Design review of the part shown in the three views and the two pictorial views. Dimensions are in mm from the part's minimum x, y and z. A direction names the side the tool comes from. Give positions to 0.01 mm unless a question says otherwise; leave off trailing zeros. Order: outer loops, then holes, each group sorted by start corner. A loop starts at its lowest first (then second) coordinate and runs counter-clockwise, first axis right, second up.
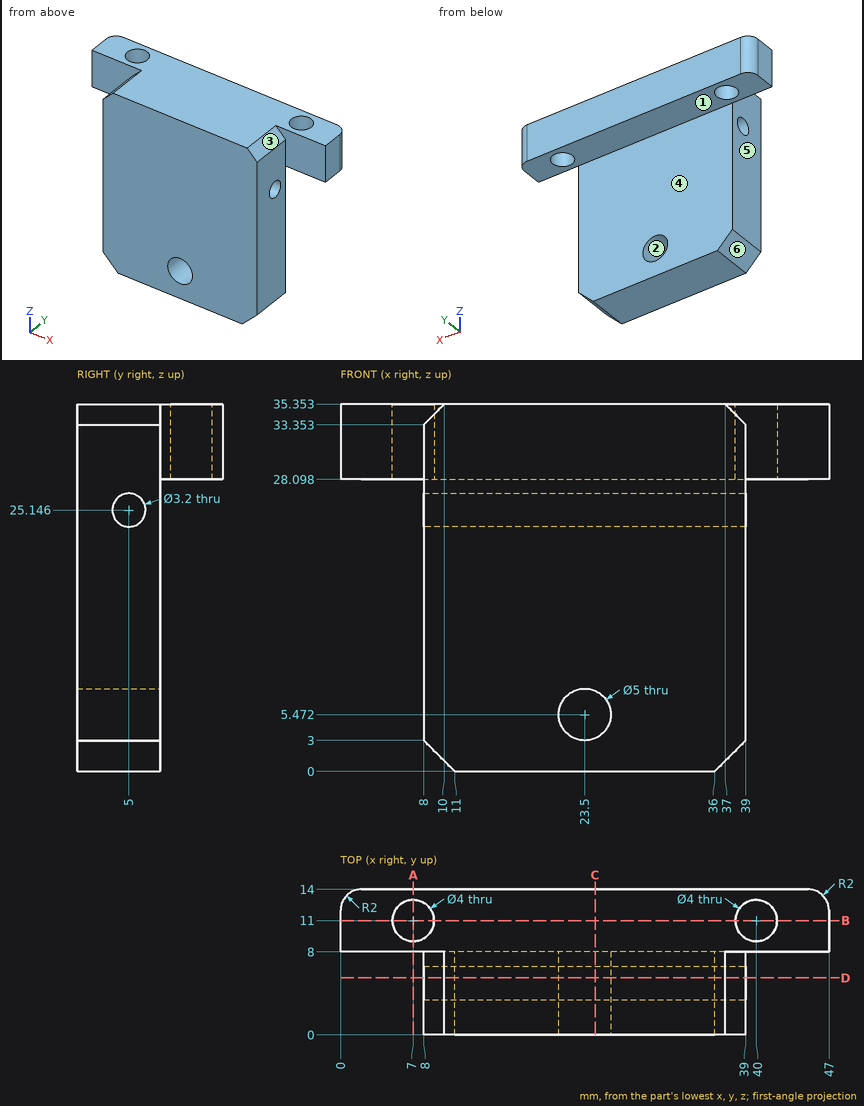
Item 1: Take a section at C-C (x = 24.5). Give the boundary of the cut face in (y, z) (1 decimal).
Values found:
outline: (0, 0) - (8, 0) - (8, 3.2) - (0, 3.2) - close; (0, 7.8) - (8, 7.8) - (8, 28.1) - (14, 28.1) - (14, 35.4) - (0, 35.4) - close; hole circle Ø3.2 at (5, 25.1)
Item 2: Take a section at D-D (y = 5.5). Give the boundary of the cut face in (x, z) (1 decimal).
Values found:
outline: (8, 3) - (11, 0) - (36, 0) - (39, 3) - (39, 23.6) - (8, 23.6) - close; (8, 26.7) - (39, 26.7) - (39, 33.4) - (37, 35.4) - (10, 35.4) - (8, 33.4) - close; hole circle Ø5 at (23.5, 5.5)
Item 3: For the marked faces 4, 5 and 6, list the 3-axis set-ups (+Z, -Z, +X, -X, +Y, -Y) from which the entire face can be reached by the end or side of a thin tool; tool diameter is ignored.
Values found:
face 4: -Z, +X, -X, +Y
face 5: +Z, -Z, -X, -Y
face 6: -Z, -X, +Y, -Y
Item 4: Take a section at A-A (x = 7). Give the boundary of the cut face in (y, z), and give its area (3 significant figures).
Values found:
outline: (8, 28.1) - (9, 28.1) - (9, 35.35) - (8, 35.35) - close; (13, 28.1) - (14, 28.1) - (14, 35.35) - (13, 35.35) - close
area: 14.5 mm2
Item 5: Take a section at B-B (y = 11). Give the boundary of the cut face in (x, z), and give its area (3 significant figures).
Values found:
outline: (0, 28.1) - (5, 28.1) - (5, 35.35) - (0, 35.35) - close; (9, 28.1) - (38, 28.1) - (38, 35.35) - (9, 35.35) - close; (42, 28.1) - (47, 28.1) - (47, 35.35) - (42, 35.35) - close
area: 283 mm2
Item 6: Draft analysis for pull direction Z (two halves, no side actions). For the marked faces 1, 2 and 3, state which applies: released by +Z, released by -Z, zero draft, split by the parting line, or undercut.
Values found:
face 1: released by -Z
face 2: undercut
face 3: released by +Z
Item 7: For line 1 (X direction, y = 11, z = 31); line 2 (Y direction, x = 7, z = 32.5); line 3 (Z direction, x = 23.5, y = 6) (1 decimal), list the stretches that pass through material, from the lowest coordinate up.
Values found:
line 1: x = 0 to 5, 9 to 38, 42 to 47
line 2: y = 8 to 9, 13 to 14
line 3: z = 0 to 3, 8 to 23.9, 26.4 to 35.4
Item 8: Clearance check with flat-ended pins moving along their axes: pin 1 Ø4 at (y, z) = (5, 25.146) entering from -X; pin 2 Ø2.5 at (x, y) = (40, 11) entering from +Z; pin 3 Ø1.8 at (x, y) = (23, 11) entering from -Z; pin 4 Ø1 at (x, y) = (38.5, 5.5) entering from -Z. State where each tip first meets the part, or that it passes through.
Values found:
pin 1: stops at x = 8
pin 2: passes through
pin 3: stops at z = 28.1
pin 4: stops at z = 2
